Can you work these out from the model? Positions are in its coordinate system, mm. Face numbers are marked on the shaded views. A direction names the side the tool comes from. Round coordinates to 2 decimals unless told otherwise and drop trailing zeros. Write each loop counter-clockwise with the first axis right and the second up, starting at its lowest first coordinate (ties: lowest second). Pieces come first, ordered by that corner, then holes. Notation, with made-up numbers: M 53.25,1.5 L 109.25,1.5 A16 ccw 109.25,31.5 Z; hole C 70.5,-7 d9. An arc over 180 degrees is marked long. Answer as a JSON object with one key per item and string values. Group by question number.
1) On a 3-axis mill with a long thin cutter (end or side, diameter ignored), from which of +Z, -Z, +X, -X, +Y, -Y can I reach the whole of each face in a straight line? I mean the marked faces 4 and 5. Say none if no direction works.
2) Suppose I cut it at B-B, the plane z = -2. Write out the boundary of the cut face in (x, y).
3) If we mould it in two halves opening along X, with no side actions, what happens to the marked faces 1, 2 and 3? For each: +X half, -X half, draft (parallel to the pull), parting line (faces both ways), or undercut.
4) I'm going to push flat-ended pins straight in: pin 1 Ø1.2 at (y, z) = (0, 3) entering from +X; pin 2 Ø0.7 at (y, z) = (0, 3) entering from -X; pin 3 Ø3 at (y, z) = (-2, 3) entering from +X. Where does each tip first touch, or does it pass through?
5) Please list where these lines run through material, in increasing order: L1, parallel to Y at x = -0.5, z = 0.75; L2, parallel to Z at x = 0, y = 0; L3, parallel to X at y = 0, z = 0. Write a range as [from, to].
6) Suppose I cut it at A-A, the plane z = 1.75. Write out the boundary of the cut face in (x, y), and give its area (3 significant figures).
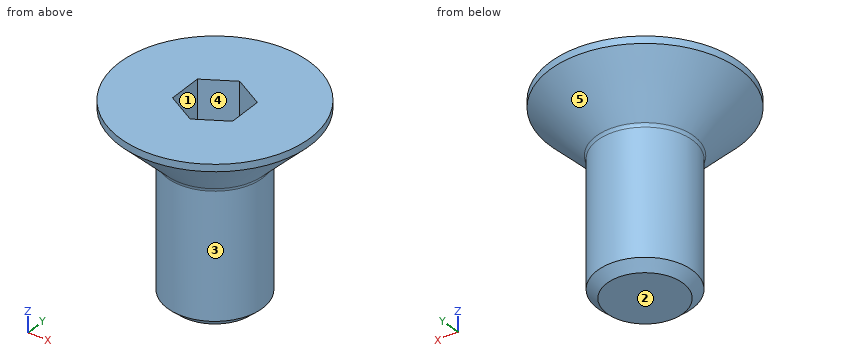
Autodesk Fusion 360 part; units mm, degrees
sketch "Sketch1" plane through (0, 0, 0) normal (0, 1, 0) x (1, 0, 0)
  line L0 (0, -4.3) -> (-4, -4.3)
  line L1 (-4, -4.3) -> (-4, -4)
  line L2 (-4, -4) -> (-2, -2)
  line L3 (-2, -2) -> (-2, 3.7)
  line L4 (-2, -2) -> (0, 0) construction
  line L5 (-2, 3.7) -> (0, 3.7)
  line L6 (0, 3.7) -> (0, -4.3)
  dimension "d5" = 45
  dimension "d9" = 4
  dimension "d10" = 8
  dimension "d72" = 2.3
  dimension "d73" = 8
revolve "Revolve1" add sketch "Sketch1" angle 360 about axis through (0, 0, -3.7) along (0, 0, 1)
sketch "Sketch6" plane through (0, 0, 4.3) normal (0, 0, 1) x (1, 0, 0)
  circle A0 centre (0, 0) radius 4
  line L0 (-1.25, 0) -> (1.25, 0) construction
  line L1 (-1.25, -0.7217) -> (-1.25, 0.7217)
  line L2 (-1.25, 0.7217) -> (0, 0)
  line L3 (-1.25, -0.7217) -> (0, 0)
  dimension "d65" = 2.5
  dimension "d67" = 60
extrude "Extrude1" cut sketch "Sketch6" against normal blind 1.8 contours L1 L2 L3
pattern_circular "C-Pattern1" count 6 over 360 about axis through (0, 0, 1.75) along (0, 0, 1) of "Extrude1"
extrude "Extrude2" cut 1 faces at (-0.4167, -0.2406, 2.5) along direction (0, 0, -1) blind 1.8
fillet "Fillet6" radius 0.2 1 edges at (-1.8647, 0.7232, 2)
thread "Thread2" thread offset 0 thread length 4.3
sketch "Sketch8" plane through (0, 0, 0) normal (0, 1, 0) x (1, 0, 0)
  line L0 (-4, -4.3) -> (-4, -4)
  line L1 (-4, -4) -> (-2, -2)
  line L2 (0, 3.7) -> (0, -4.3)
  line L3 (0, -4.3) -> (-4, -4.3)
  line L4 (0, 3.7) -> (-2.04, 3.7)
  line L5 (-2.04, 3.7) -> (-2.04, 3.3)
  line L6 (-2.04, 3.3) -> (-1.6, 3.7)
  dimension "d104" = 1.6
  dimension "d106" = 2.04
  dimension "d107" = 0.4
revolve "Revolve3" cut sketch "Sketch8" angle 360 about axis through (0, 0, -3.7) along (0, 0, 1)
equation "d5 = adsk_headang * 0.5"
equation "d9 = adsk_nomdia"
equation "d10 = adsk_nomlen"
equation "adsk_nomlen = 8.00 mm"
equation "adsk_headh = 2.30 mm"
equation "adsk_headdia = 8.00 mm"
equation "adsk_nomdia = 4.00 mm"
equation "adsk_headang = 90.00 deg"
equation "adsk_philwidth = 2.50 mm"
equation "adsk_phildepth = 1.80 mm"
equation "d65 = adsk_philwidth"
equation "d72 = adsk_headh"
equation "d73 = adsk_headdia"
equation "d77 = adsk_thrlen"
equation "adsk_thrlen = 4.30 mm"
equation "adsk_midfillet = 0.20 mm"
equation "d85 = adsk_midfillet"
equation "adsk_startlen = adsk_nomdia * 0.1"
equation "adsk_startang = 45 deg"
equation "d99 = ( adsk_nomdia / 2 ) * tan(90 deg - adsk_headang / 2) + adsk_headh"
equation "adsk_endpointdia = adsk_nomdia - 2 * adsk_startlen"
equation "d104 = adsk_endpointdia / 2"
equation "d106 = adsk_nomdia * 0.51"
equation "d107 = adsk_startlen"
properties part number "arrangementsContainer"
Results:
{
 "1": {"face 4": "+Z", "face 5": "-Z"},
 "2": {"outline": "C 0,0 d4"},
 "3": {"face 1": "undercut", "face 2": "draft", "face 3": "parting line"},
 "4": {"pin 1": "x = 3.6", "pin 2": "x = -3.35", "pin 3": "x = 3.9"},
 "5": {"L1": "[-1.94, -1.15], [1.15, 1.94]", "L2": "[-3.7, 0.7]", "L3": "[-2, 2]"},
 "6": {"outline": "C 0,0 d4; hole M -1.25,-0.72 L 0,-1.44 L 1.25,-0.72 L 1.25,0.72 L 0,1.44 L -1.25,0.72 Z", "area": "7.15 mm^2"}
}
